from build123d import *

# Parameters (mm, degrees)
F0_W      = 12.7
F0_H      = 12.7
F1_DEPTH  = 12.7
F3_DEPTH  = 12.7
F3_FACE_W = 12.7
F3_FACE_H = 19.05


with BuildPart() as f1:
    # F0 (on Top) → F1 (new body)
    with BuildSketch(Plane.XY):
        with Locations((-42.6943581551, 29.7822718922)):
            Rectangle(F0_W, F0_H)
    extrude(amount=F1_DEPTH)

    # F2 (on face) → F3 (join)
    with BuildSketch(Plane.YZ.offset(-36.3443581551)):
        Polygon((17.7597312508, 12.7), (23.4322718922, 12.7), (36.1322718922, 12.7), (41.2083510732, 12.7), (29.484041162, 27.714761307), align=None)
    extrude(amount=-F3_DEPTH)

    # F4: sweep along a path in F4_path
    with BuildLine(Plane(origin=(-49.0443581551, 29.484041162, 27.714761307), x_dir=(0, -0.6154493392, 0.7881764466), z_dir=(0, -0.7881764466, -0.6154493392))) as f4_path:
        Line((0, 0), (-19.05, 0))
    # F3_face (on face) → F4 (sweep)
    with BuildSketch(Plane(origin=(-42.6943581551, 23.6218862064, 20.2073806535), x_dir=(1, 0, 0), z_dir=(0, -0.7881764466, 0.6154493392))):
        Rectangle(F3_FACE_W, F3_FACE_H)
    sweep(path=f4_path.line)


solid = f1.part
Model file for the job. Use its own axes, mm. A direction names the side the tool comes from. Give positions to 0.01 mm unless a question says otherwise; leave off trailing zeros. Order: outer loops, then holes, each group sorted by start corner. A loop starts at its lowest first (then second) coordinate and runs counter-clockwise, first axis right, second up. Notation, with made-up numbers: (-18.75, -38.5) - (-10.75, -38.5) arc R24 ccw to (-10.75, -28.5) - close; hole circle Ø9 at (68, 47.5). An arc over 180 degrees is marked (long way). One line per item, written item: value.
Item 1: Slice it at B-B (y = 30.5). List the corners of the cut face in (x, z), then the cut area to 3 significant figures.
Response values:
outline: (-49.04, -1.01) - (-36.34, -1.01) - (-36.34, 26.41) - (-49.04, 26.41) - close
area: 348 mm2
Item 2: Wall check: line 1 (Y direction, x = -38.25, z = 3); line 2 (Y direction, x = -48, z = 14); line 3 (Z direction, x = -45.5, y = 38.25). Give the ranges that are in metal, low to high.
Response values:
line 1: 23.43 to 36.13
line 2: 18.77 to 40.19
line 3: 8.91 to 16.49
Item 3: Slice it at A-A (x = -42). List the corners of the cut face in (y, z), then the cut area to 3 significant figures.
Response values:
outline: (17.76, 12.7) - (23.43, 5.44) - (23.43, 0) - (27.68, 0) - (29.48, -2.31) - (31.29, 0) - (36.13, 0) - (36.13, 6.2) - (41.21, 12.7) - (29.48, 27.71) - close
area: 379 mm2
Item 4: Pin check, flat tips, straight feed: pin 1 Ø3 at (x, y) = (-45, 27) entering from +Z; pin 2 Ø2 at (x, z) = (-40, 1.5) entering from -Y; pin 3 Ø4 at (x, y) = (-43.5, 35) entering from -Z. Stop position of each tip, or through.
Response values:
pin 1: z = 26.45
pin 2: y = 23.43
pin 3: z = 0
Item 5: Tool access for faces 1 (the flat face through (-43, 26, 0)), 2 (the flat face through (-43, 36.132, 3)), 3 (the flat face through (-42.61, 35.43, 20.1)): list every direction of +Z, -Z, +X, -X, +Y, -Y with a clear straight run to the whole face (end or side of a thin tool).
Response values:
face 1: -Z, +X, -X, -Y
face 2: -Z, +X, -X, +Y
face 3: +Z, +X, -X, +Y
Item 6: Slice it at C-C (z = 17). List the corners of the cut face in (x, y).
Response values:
outline: (-49.04, 21.12) - (-36.34, 21.12) - (-36.34, 37.85) - (-49.04, 37.85) - close
Item 7: Two-plate mould, pull along Z, no slides. Class faces 4 (the flat face through (-36.344, 29, 13)), 5 (the flat face through (-42.61, 23.7, 20.31)), 6 (the flat face through (-42.78, 28.59, -1.17)): released by +Z, released by -Z, zero draft, split by the parting line, or undercut.
Response values:
face 4: zero draft
face 5: released by +Z
face 6: released by -Z
